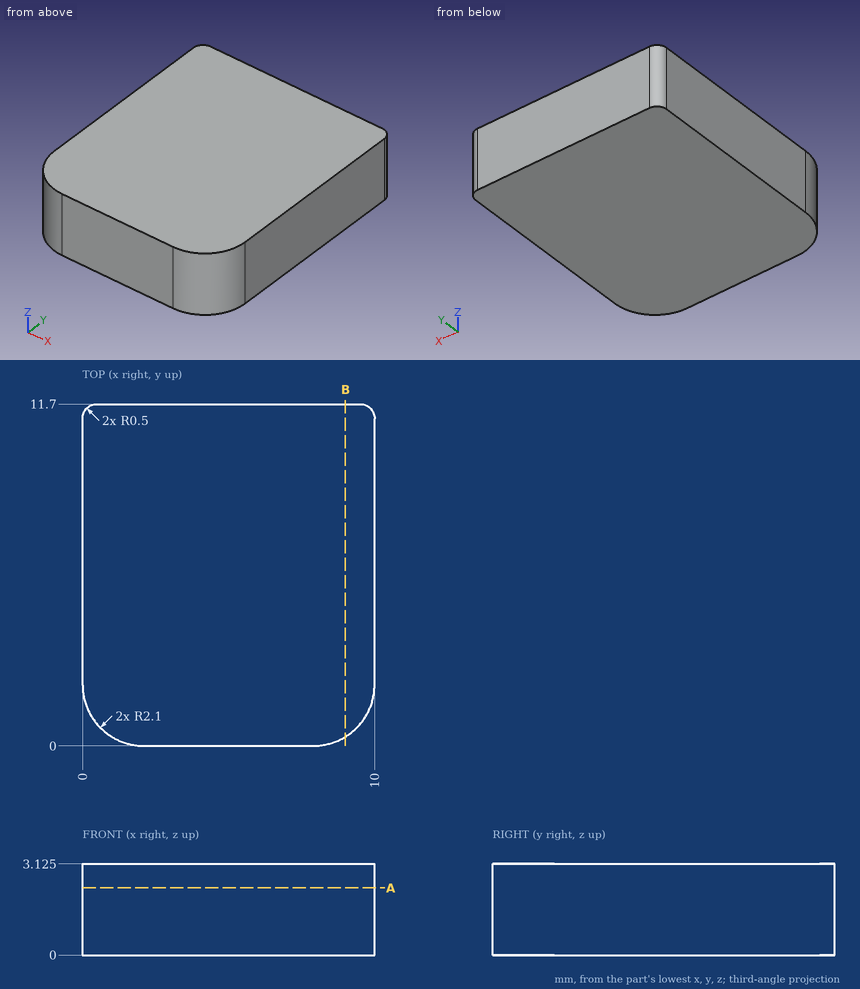
Geometry: see drawing. Coordinates: mm, zero at the bounding-box minimum. Round coordinates to 2 decimals unless told otherwise and drop trailing zeros. Loops run counter-clockwise (first coordinate to the right, second up) from the corner with the lowest first, then second, coordinate; pieces in that order, holes last. Notation, with made-up numbers: M 41.5,15.25 L 50.5,15.25 A23 cw 50.5,46.25 Z; hole C 11.25,18.25 d11. An arc over 180 degrees is marked long. Use a Markdown table: item, result. Add a question column.
1. Section query B-B on x = 9. Return the cut outline in (y, z) (3 decimals).
2. Line query: line 1 (Y direction, x = 2, z = 2.15); line 2 (X direction, y = 1, z = 0.15); line 3 (Y direction, x = 9, z = 2.85). Output: solid intervals per line, ascending.
3. Section query A-A on z = 2.3. Return the cut outline in (x, y).
Reported:
| question | item | result |
|---|---|---|
| 1 | outline | M 0.311,0 L 11.7,0 L 11.7,3.125 L 0.311,3.125 Z |
| 2 | line 1 | y = 0 to 11.7 |
| 2 | line 2 | x = 0.31 to 9.69 |
| 2 | line 3 | y = 0.31 to 11.7 |
| 3 | outline | M 0,2.1 A2.1 ccw 2.1,0 L 7.9,0 A2.1 ccw 10,2.1 L 10,11.2 A0.5 ccw 9.5,11.7 L 0.5,11.7 A0.5 ccw 0,11.2 Z |
